from build123d import *

# Parameters (mm, degrees)
BOSS_EXTRUDE1_DEPTH = 100
SKETCH2_W           = 120
SKETCH2_H           = 100
BOSS_EXTRUDE2_DEPTH = 92
SKETCH3_R           = 4.5
CUT_EXTRUDE1_DEPTH  = 85
SKETCH4_R           = 2.65
CUT_EXTRUDE2_DEPTH  = 7
CUT_EXTRUDE3_REACH  = 159.053
FILLET1_R           = 100
FILLET2_R           = 100
FILLET4_R           = 10
FILLET5_R           = 5


with BuildPart() as part:
    # Sketch1 → Boss-Extrude1 (new body)
    with BuildSketch(Plane.XY):
        Polygon((0, 0), (-37.5, 0), (-37.5, 40), (-27.5, 40), (-27.5, 10), (-10, 10), (-10, 40), (0, 40), align=None)
    extrude(amount=BOSS_EXTRUDE1_DEPTH)

    # Sketch2 → Boss-Extrude2 (add)
    with BuildSketch(Plane.XZ):
        with Locations((-18.75, 50)):
            Rectangle(SKETCH2_W, SKETCH2_H)
    extrude(amount=BOSS_EXTRUDE2_DEPTH)

    # Sketch3 → Cut-Extrude1 (cut)
    with BuildSketch(Plane(origin=(0, 0, 0), x_dir=(1, 0, 0), z_dir=(0, 1, 0))):
        with Locations(Location((26.25, -50, 0), (0, 0, 180))):
            Circle(SKETCH3_R)
        with Locations(Location((-63.75, -50, 0), (0, 0, 180))):
            Circle(SKETCH3_R)
    extrude(amount=-CUT_EXTRUDE1_DEPTH, mode=Mode.SUBTRACT)

    # Sketch4 → Cut-Extrude2 (cut)
    with BuildSketch(Plane(origin=(0, -85, 0), x_dir=(1, 0, 0), z_dir=(0, 1, 0))):
        with Locations(Location((26.25, -50, 0), (0, 0, 180))):
            Circle(SKETCH4_R)
        with Locations(Location((-63.75, -50, 0), (0, 0, 180))):
            Circle(SKETCH4_R)
    extrude(amount=-CUT_EXTRUDE2_DEPTH, mode=Mode.SUBTRACT)

    # Cut-Extrude3: up to this face of the body (flat: up to its plane)
    cut_extrude3_end = Plane(part.part.faces().sort_by_distance((-18.75, -40.86267166, 100))[0])
    # Sketch5 → Cut-Extrude3 (cut, up to the picked face)
    with BuildSketch(Plane(origin=(0, 0, 0), x_dir=(-1, 0, 0), z_dir=(0, 0, -1)), mode=Mode.PRIVATE) as cut_extrude3_sk1:
        Polygon((0, 0), (-41.25, -80), (-41.25, 0), align=None)
    cut_extrude3_tool1 = split(extrude(cut_extrude3_sk1.sketch, amount=-CUT_EXTRUDE3_REACH, mode=Mode.PRIVATE), bisect_by=cut_extrude3_end, keep=Keep.BOTH, mode=Mode.PRIVATE)
    # Sketch5 → Cut-Extrude3 (cut, up to the picked face)
    with BuildSketch(Plane(origin=(0, 0, 0), x_dir=(-1, 0, 0), z_dir=(0, 0, -1)), mode=Mode.PRIVATE) as cut_extrude3_sk2:
        Polygon((37.5, 0), (78.75, 0), (78.75, -80), align=None)
    cut_extrude3_tool2 = split(extrude(cut_extrude3_sk2.sketch, amount=-CUT_EXTRUDE3_REACH, mode=Mode.PRIVATE), bisect_by=cut_extrude3_end, keep=Keep.BOTH, mode=Mode.PRIVATE)
    add(cut_extrude3_tool1.solids().sort_by(Axis((27.5, -26.666667, 0), (0, 0, 1)))[0], mode=Mode.SUBTRACT)
    add(cut_extrude3_tool2.solids().sort_by(Axis((-65, -26.666667, 0), (0, 0, 1)))[0], mode=Mode.SUBTRACT)

    # Fillet1
    fillet1_edges = [part.edges().sort_by_distance(p)[0] for p in [
        (0, 0, 50),
    ]]
    fillet(fillet1_edges, radius=FILLET1_R)

    # Fillet2
    fillet2_edges = [part.edges().sort_by_distance(p)[0] for p in [
        (-37.5, 0, 50),
    ]]
    fillet(fillet2_edges, radius=FILLET2_R)

    # Fillet4
    fillet4_edges = [part.edges().sort_by_distance(p)[0] for p in [
        (-37.5, 32.131733499, 100),
        (-40.319673611, 0.684150576, 100),
        (-37.5, 32.131733499, 0),
        (-40.319673611, 0.684150576, 0),
        (-63.68484163, -50.78272316, 100),
        (-63.68484163, -50.78272316, 0),
        (0, 32.131733499, 0),
        (2.819673611, 0.684150576, 0),
        (0, 32.131733499, 100),
        (2.819673611, 0.684150576, 100),
        (26.18484163, -50.78272316, 0),
        (26.18484163, -50.78272316, 100),
        (41.25, -86, 0),
        (41.25, -86, 100),
        (-78.75, -86, 100),
        (-78.75, -86, 0),
    ]]
    fillet(fillet4_edges, radius=FILLET4_R - 0.0001)  # a hair under: the kernel refuses the full size

    # Fillet5
    fillet5_edges = [part.edges().sort_by_distance(p)[0] for p in [
        (-37.5, 40, 50),
        (-34.571097101, 40, 97.071097101),
        (-34.571097101, 40, 2.928902899),
        (0, 40, 50),
        (-2.928902899, 40, 97.071097101),
        (-2.928902899, 40, 2.928902899),
    ]]
    fillet(fillet5_edges, radius=FILLET5_R)


solid = part.part
Here's how the part is built. I have some questions about the finished solid (model axes, mm). A direction names the side the tool comes from. Round coordinates to 2 decimals unless told otherwise and drop trailing zeros. Write each loop counter-clockwise with the first axis right and the second up, starting at its lowest first coordinate (ties: lowest second). Pieces come first, ordered by that corner, then holes. Notation, with made-up numbers: (31.25, -20) -> (77.25, -20) arc R27 ccw to (77.25, 18) -> close; hole circle Ø2 at (-37.5, 22.5). An arc over 180 degrees is marked (long way). One line per item, written item: value.
1) For faces 1 (the face through (-66, -85, 48)), 2 (the face through (-37.5, 30, 49)), 3 (the face through (-34.49, 29.71, 97.15)), 4 (the face through (38.4, -86.08, 3.01)), 5 (the face through (23.72, -52.57, 97.15)), which set-ups out of +Z, -Z, +X, -X, +Y, -Y let a thin tool reach every point of the face, with its end or its side?
Filled sheet:
face 1: +Y
face 2: +Z, -Z, -X, +Y
face 3: +Z, -X, +Y
face 4: -Z, +X, +Y, -Y
face 5: +Z, +X, +Y
2) We'd pull the mould along X, two halves only. Please class faces 6 (the face through (0, 30, 49)), 7 (the face through (-34.65, 29.71, 3.01)), 8 (the face through (-27.5, 25, 49)): released by +X, released by -X, zero draft, split by the parting line, or undercut.
Filled sheet:
face 6: released by +X
face 7: released by -X
face 8: undercut
3) Suppose I cut it at C-C on z = 67. List the corners of the cut face in (x, y) for me, plus the area to 3 significant figures.
Filled sheet:
outline: (-78.75, -92) -> (41.25, -92) -> (41.25, -80) -> (11.12, -21.57) arc R100 cw to (0, 24.26) -> (0, 35) arc R5 ccw to (-5, 40) -> (-10, 40) -> (-10, 10) -> (-27.5, 10) -> (-27.5, 40) -> (-32.5, 40) arc R5 ccw to (-37.5, 35) -> (-37.5, 24.26) arc R100 cw to (-48.62, -21.57) -> (-78.75, -80) -> close
area: 8,800 mm2
4) Suppose I cut it at B-B on z = 50. Give the number of separate pieces and of enclosed holes in the cut face, plus the area to 3 significant figures.
Filled sheet:
separate pieces: 3
enclosed holes: 0
area: 8,110 mm2
5) If I drill on line 1 (Z direction, x = -63.75, y = -88); line 2 (Z direction, x = -63.75, y = -75); line 3 (X direction, y = -75, z = 50), over which ranges is the centre line in solid material (lowest first)? Write a range as [from, to].
Filled sheet:
line 1: z = [0, 47.35], [52.65, 100]
line 2: z = [0, 45.5], [54.5, 100]
line 3: x = [-76.17, -68.25], [-59.25, 21.75], [30.75, 38.67]
6) I'm going to push flat-ended pins straight in: pin 1 Ø6 at (y, z) = (-47.5, 47.5) entering from -X; pin 2 Ø7 at (x, z) = (26.25, 50) entering from +Y; pin 3 Ø8.5 at (y, z) = (29, 30.5) entering from +X. Where does each tip first touch, or does it pass through?
Filled sheet:
pin 1: stops at x = -63.16
pin 2: stops at y = -85
pin 3: stops at x = 0
